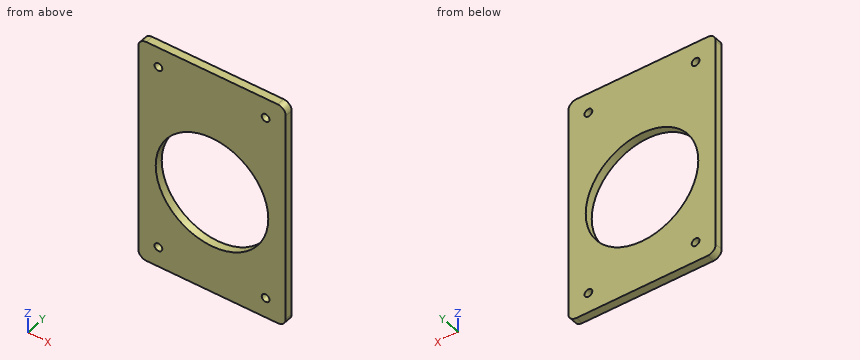
```python
from build123d import *

# Parameters (mm, degrees)
SKETCH_1_W          = 55
SKETCH_1_H          = 85
SKETCH_1_R          = 21
EXTRUDE_1_DEPTH     = 3
SKETCH_2_R          = 1.45
CUT_EXTRUDE_1_DEPTH = 3
FILLET_1_R          = 3


with BuildPart() as part:
    # 草图1 → 凸台-拉伸1 (new body)
    with BuildSketch(Plane(origin=(0, 0, 0), x_dir=(1, 0, 0), z_dir=(0, 1, 0))):
        with Locations((0, -3.75)):
            Rectangle(SKETCH_1_W, SKETCH_1_H)
        with Locations(Location((0, 0, 0), (0, 0, 270))):
            Circle(SKETCH_1_R, mode=Mode.SUBTRACT)
    extrude(amount=EXTRUDE_1_DEPTH)

    # 草图2 → 切除-拉伸1 (cut)
    with BuildSketch(Plane(origin=(0, 3, 0), x_dir=(1, 0, 0), z_dir=(0, 1, 0))):
        with Locations(Location((-20, 31.25, 0), (0, 0, 270))):
            Circle(SKETCH_2_R)
        with Locations(Location((20, 31.25, 0), (0, 0, 270))):
            Circle(SKETCH_2_R)
        with Locations(Location((-20, -38.75, 0), (0, 0, 90))):
            Circle(SKETCH_2_R)
        with Locations(Location((20, -38.75, 0), (0, 0, 90))):
            Circle(SKETCH_2_R)
    extrude(amount=-CUT_EXTRUDE_1_DEPTH, mode=Mode.SUBTRACT)

    # 圆角1
    fillet_1_edges = [part.edges().sort_by_distance(p)[0] for p in [
        (27.5, 1.5, 46.25),
        (-27.5, 1.5, 46.25),
        (-27.5, 1.5, -38.75),
        (27.5, 1.5, -38.75),
    ]]
    fillet(fillet_1_edges, radius=FILLET_1_R)


solid = part.part
```
Input: part model. Units: mm. Frame: model coordinates. Round coordinates to 2 decimals unless told otherwise and drop trailing zeros. Loops run counter-clockwise (first coordinate to the right, second up) from the corner with the lowest first, then second, coordinate; pieces in that order, holes last. Notation, with made-up numbers: M -12,24.5 L 2,24.5 A10 ccw 2,42.5 Z; hole C 9.25,5.5 d8. An arc over 180 degrees is marked long. Answer in a Markdown table with one row per item. Add a question column.
1. Section A-A (z = -31.25). Output: boundary loops of the cut face in (x, y).
2. Section C-C (z = 0). Output: boundary loops of the cut face in (x, y), and give its area (3 significant figures).
3. Ray query, probe 1 along X at (y, z) = (1.7, -31.25); probe 2 along X at (y, z) = (2.05, 0); probe 3 along Z at (x, y) = (3, 1.7). Return the intervals inside material, ascending.
4. Section B-B (y = 2.4). Output: boundary loops of the cut face in (x, z).
5. Contact query for a flat-ended pin moving along its axis: pin 1 (1.7 mm diameter, centred on x = -20, z = 38.75, fed in from +Y). Output: stop coordinate, or through.
6. Section D-D (x = 12.5). Output: boundary loops of the cut face in (y, z), and give its area (3 significant figures).
Values follow:
| question | item | result |
|---|---|---|
| 1 | outline | M -27.5,0 L -21.45,0 L -21.45,3 L -27.5,3 Z; M -18.55,0 L 18.55,0 L 18.55,3 L -18.55,3 Z; M 21.45,0 L 27.5,0 L 27.5,3 L 21.45,3 Z |
| 2 | outline | M -27.5,0 L -21,0 L -21,3 L -27.5,3 Z; M 21,0 L 27.5,0 L 27.5,3 L 21,3 Z |
| 2 | area | 39.0 mm^2 |
| 3 | probe 1 | -27.5 to -21.45, -18.55 to 18.55, 21.45 to 27.5 |
| 3 | probe 2 | -27.5 to -21, 21 to 27.5 |
| 3 | probe 3 | -38.75 to -20.78, 20.78 to 46.25 |
| 4 | outline | M -27.5,-35.75 A3 ccw -24.5,-38.75 L 24.5,-38.75 A3 ccw 27.5,-35.75 L 27.5,43.25 A3 ccw 24.5,46.25 L -24.5,46.25 A3 ccw -27.5,43.25 Z; hole C -20,-31.25 d2.9; hole C -20,38.75 d2.9; hole C 0,0 d42; hole C 20,-31.25 d2.9; hole C 20,38.75 d2.9 |
| 5 | pin 1 | through |
| 6 | outline | M 0,-38.75 L 3,-38.75 L 3,-16.87 L 0,-16.87 Z; M 0,16.87 L 3,16.87 L 3,46.25 L 0,46.25 Z |
| 6 | area | 154 mm^2 |
